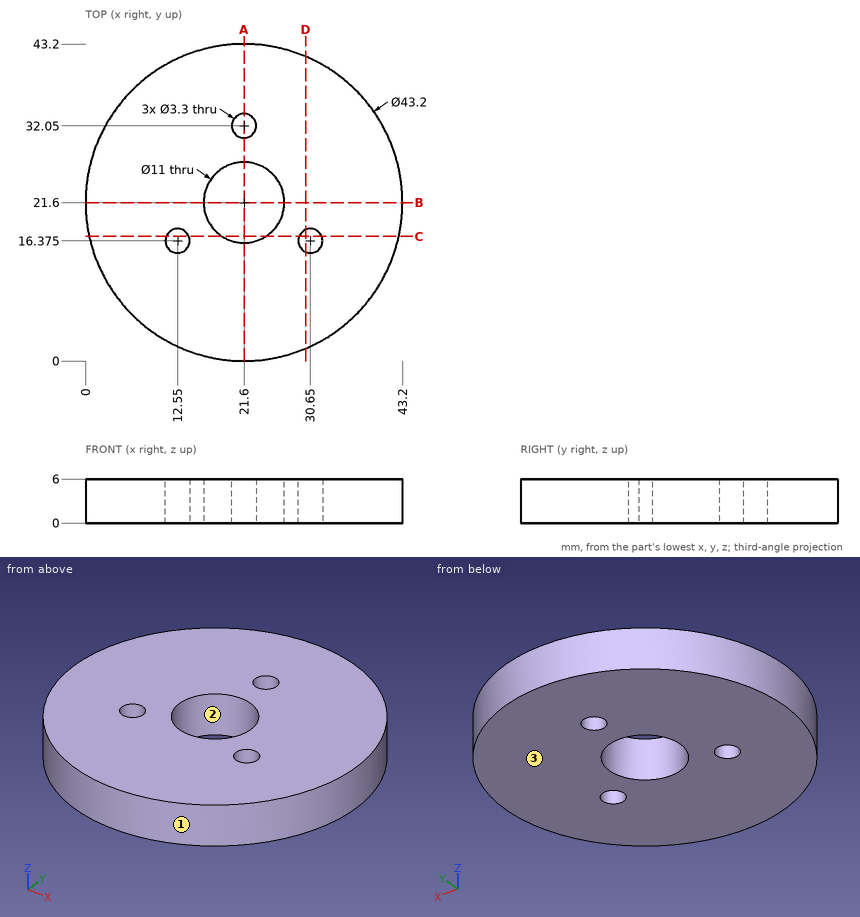
Study the drawing (mm; zero at the part's minimum x, y, z) and answer. Give positions to 0.01 mm unless a question says otherwise; leave off trailing zeros. Loops run counter-clockwise (first coordinate to the right, second up) from the corner with the lowest first, then second, coordinate; pieces in that order, holes last. Notation, with made-up numbers: (67.25, -5) - (124.25, -5) arc R7 cw to (124.25, 2) - close; hole circle Ø3 at (8.5, 73). An arc over 180 degrees is marked (long way). Answer in a Markdown table with one row per item. Add a question column.
Q1. The part is cut by section D-D (x = 30). Determine the outline of the cut face in (y, z).
Q2. Consider line 1 along Y through (x, z) = (21.6, 4.15); line 2 along X through (y, z) = (15, 5.45); line 3 along X through (y, z) = (21, 4.3). Determine where each line is inside the solid, lowest interval first.
Q3. The part is cut by section C-C (y = 17). Determine the outline of the cut face in (x, z) (1 decimal).
Q4. The part is cut by section B-B (y = 21.6). Determine the outline of the cut face in (x, z).
Q5. The part is cut by section A-A (x = 21.6). Determine the outline of the cut face in (y, z), and give its area (3 significant figures).
Q6. Determine the mould class of the marked faces 1, 2 and 3 for opening direction Y: released by +Y, released by -Y, zero draft, split by the parting line, or undercut.
Q7. Each of these flat-tipped pins is pushed along its axis until it touches: P1, Ø4.5, axis at x = 12.55, y = 16.38, coming from the -Z side; P2, Ø2, axis at y = 24.5, z = 5.5, coming from the -X side. Where does it stop, or does it pass through?
Solution:
| question | item | result |
|---|---|---|
| 1 | outline | (1.7, 0) - (14.86, 0) - (14.86, 6) - (1.7, 6) - close; (17.89, 0) - (41.5, 0) - (41.5, 6) - (17.89, 6) - close |
| 2 | line 1 | y = 0 to 16.1, 27.1 to 30.4, 33.7 to 43.2 |
| 2 | line 2 | x = 1.03 to 11.64, 13.46 to 29.74, 31.56 to 42.17 |
| 2 | line 3 | x = 0.01 to 16.13, 27.07 to 43.19 |
| 3 | outline | (0.5, 0) - (11, 0) - (11, 6) - (0.5, 6) - close; (14.1, 0) - (18.6, 0) - (18.6, 6) - (14.1, 6) - close; (24.6, 0) - (29.1, 0) - (29.1, 6) - (24.6, 6) - close; (32.2, 0) - (42.7, 0) - (42.7, 6) - (32.2, 6) - close |
| 4 | outline | (0, 0) - (16.1, 0) - (16.1, 6) - (0, 6) - close; (27.1, 0) - (43.2, 0) - (43.2, 6) - (27.1, 6) - close |
| 5 | outline | (0, 0) - (16.1, 0) - (16.1, 6) - (0, 6) - close; (27.1, 0) - (30.4, 0) - (30.4, 6) - (27.1, 6) - close; (33.7, 0) - (43.2, 0) - (43.2, 6) - (33.7, 6) - close |
| 5 | area | 173 mm² |
| 6 | face 1 | split by the parting line |
| 6 | face 2 | undercut |
| 6 | face 3 | zero draft |
| 7 | P1 | stops at z = 0 |
| 7 | P2 | stops at x = 0.08 |
